Could you check a few things on this model? Use its own coordinates, in mm. A direction names the side the tool comes from. Give positions to 0.01 mm unless a question says otherwise; leave off trailing zeros. Loops run counter-clockwise (first coordinate to the right, second up) from the corner with the lowest first, then second, coordinate; pieces in that order, holes last. Notation, with made-up numbers: M -9.75,36.25 L 49.25,36.25 A17 cw 49.25,54.25 Z; hole C -29.75,49 d2. An arc over 180 degrees is marked long. Use a Markdown table: item, result. Add a question column.
1) If I drill on line 1 along Y through (x, z) = (-33.5, 4.5); line 2 along X through (y, z) = (-18, 13.5); line 3 along Z through (x, y) = (-14, -39), over which ranges is the centre line in solid material (lowest first)? Write a range as [from, to].
2) Suppose I cut it at B-B on y = 9.5. List the corners of the cut face in (x, z) for me, and give its area (3 significant figures).
3) Suppose I cut it at C-C on z = 15.5. List the corners of the cut face in (x, y) for me, and give its area (3 significant figures).
4) We'd pull the mould along X, two halves only. Please class faces 4 (the flat face through (-39.643, -16, 13)), 5 (the flat face through (-39, -15, 25.4)), 6 (the cylindrical face through (-17.73, 25.418, 10.244)): +X half, -X half, draft (parallel to the pull), parting line (faces both ways), or undercut.
5) Will this pin go through, and if not, where does the flat tip stop? pin 1 Ø10 at (x, y) = (14, 4.5) entering from -Z.
6) Suppose I cut it at A-A on z = 22.75. List the corners of the cut face in (x, y) for me.
7) Which directions (+Z, -Z, +X, -X, +Y, -Y) give clear straight access to the entire face, cutting with the end or side of a thin tool? Please do faces 1 (the flat face through (21.317, -16, 13)), 2 (the flat face through (-22, -56, 7.239)), 3 (the flat face through (-10, -54.61, 14)).
8) Suppose I cut it at D-D on x = 11. List the corners of the cut face in (y, z) for me.
```python
from build123d import *

# Parameters (mm, degrees)
F0_W     = 60.96
F0_H     = 83.82
F1_DEPTH = 25.4
F2_T     = -2.54
F3_W     = 13.97
F3_H     = 12.192
F4_DEPTH = 2.54
F5_R     = 5.08
F6_DEPTH = 2.54


with BuildPart() as f1:
    # F0 (on Top) → F1 (new body)
    with BuildSketch(Plane.XY):
        with Locations((-9.163326, -15.24)):
            Rectangle(F0_W, F0_H)
    extrude(amount=F1_DEPTH)

    # F2
    f2_openings = [f1.faces().sort_by_distance(p)[0] for p in [
        (-9.163326, -15.24, 25.4),
    ]]
    offset(amount=F2_T, openings=f2_openings)

    # F3 (on face) → F4 (cut, through all)
    with BuildSketch(Plane.XZ.offset(57.15)):
        with Locations((-21.482326, 13.335)):
            Rectangle(F3_W, F3_H)
    extrude(amount=-F4_DEPTH, mode=Mode.SUBTRACT)

    # F5 (on face) → F6 (cut, through all)
    with BuildSketch(Plane(origin=(0, 26.67, 0), x_dir=(-1, 0, 0), z_dir=(0, 1, 0))):
        with Locations((21.761726, 13.335)):
            Circle(F5_R)
    extrude(amount=-F6_DEPTH, mode=Mode.SUBTRACT)


solid = f1.part
```
Answer block:
| question | item | result |
|---|---|---|
| 1 | line 1 | y = [-57.15, -54.61], [24.13, 26.67] |
| 1 | line 2 | x = [-39.64, -37.1], [18.78, 21.32] |
| 1 | line 3 | z = [0, 2.54] |
| 2 | outline | M -39.64,0 L 21.32,0 L 21.32,25.4 L 18.78,25.4 L 18.78,2.54 L -37.1,2.54 L -37.1,25.4 L -39.64,25.4 Z |
| 2 | area | 271 mm^2 |
| 3 | outline | M -39.64,-57.15 L -28.47,-57.15 L -28.47,-54.61 L -37.1,-54.61 L -37.1,24.13 L -26.36,24.13 L -26.36,26.67 L -39.64,26.67 Z; M -17.17,24.13 L 18.78,24.13 L 18.78,-54.61 L -14.5,-54.61 L -14.5,-57.15 L 21.32,-57.15 L 21.32,26.67 L -17.17,26.67 Z |
| 3 | area | 651 mm^2 |
| 4 | face 4 | -X half |
| 4 | face 5 | draft |
| 4 | face 6 | undercut |
| 5 | pin 1 | stops at z = 0 |
| 6 | outline | M -39.64,-57.15 L 21.32,-57.15 L 21.32,26.67 L -39.64,26.67 Z; hole M -37.1,-54.61 L 18.78,-54.61 L 18.78,24.13 L -37.1,24.13 Z |
| 7 | face 1 | +Z, -Z, +X, +Y, -Y |
| 7 | face 2 | -Y |
| 7 | face 3 | +Z |
| 8 | outline | M -57.15,0 L 26.67,0 L 26.67,25.4 L 24.13,25.4 L 24.13,2.54 L -54.61,2.54 L -54.61,25.4 L -57.15,25.4 Z |
